```python
from build123d import *

# Parameters (mm, degrees)
BOSS_EXTRUDE1_DEPTH = 6.35
CUT_EXTRUDE1_REACH  = 8.35
SKETCH2_R           = 2.413
CUT_EXTRUDE3_REACH  = 8.35
SKETCH4_R           = 1.397
SKETCH4_R_2         = 4.7625
FILLET4_R           = 12.7
FILLET5_R           = 19.05


with BuildPart() as part:
    # Sketch1 → Boss-Extrude1 (new body)
    with BuildSketch(Plane.XY):
        Polygon((0, 0), (12.7, 0), (12.7, 50.8), (50.8, 50.8), (50.8, 0), (63.5, 0), (63.5, 69.85), (44.45, 101.6), (19.05, 101.6), (0, 82.55), align=None)
    extrude(amount=BOSS_EXTRUDE1_DEPTH)

    # Sketch2 → Cut-Extrude1 (cut, up to next)
    with BuildSketch(Plane.XY.offset(6.35), mode=Mode.PRIVATE) as cut_extrude1_sk1:
        with Locations((6.35, 12.7)):
            Circle(SKETCH2_R)
    cut_extrude1_tool1 = extrude(cut_extrude1_sk1.sketch, amount=-CUT_EXTRUDE1_REACH, mode=Mode.PRIVATE) & part.part
    add(cut_extrude1_tool1.solids().sort_by_distance((6.35, 12.7, 6.35))[0], mode=Mode.SUBTRACT)
    # Sketch2 → Cut-Extrude1 (cut, up to next)
    with BuildSketch(Plane.XY.offset(6.35), mode=Mode.PRIVATE) as cut_extrude1_sk2:
        with Locations((6.35, 31.75)):
            Circle(SKETCH2_R)
    cut_extrude1_tool2 = extrude(cut_extrude1_sk2.sketch, amount=-CUT_EXTRUDE1_REACH, mode=Mode.PRIVATE) & part.part
    add(cut_extrude1_tool2.solids().sort_by_distance((6.35, 31.75, 6.35))[0], mode=Mode.SUBTRACT)
    # Sketch2 → Cut-Extrude1 (cut, up to next)
    with BuildSketch(Plane.XY.offset(6.35), mode=Mode.PRIVATE) as cut_extrude1_sk3:
        with Locations((57.15, 12.7)):
            Circle(SKETCH2_R)
    cut_extrude1_tool3 = extrude(cut_extrude1_sk3.sketch, amount=-CUT_EXTRUDE1_REACH, mode=Mode.PRIVATE) & part.part
    add(cut_extrude1_tool3.solids().sort_by_distance((57.15, 12.7, 6.35))[0], mode=Mode.SUBTRACT)
    # Sketch2 → Cut-Extrude1 (cut, up to next)
    with BuildSketch(Plane.XY.offset(6.35), mode=Mode.PRIVATE) as cut_extrude1_sk4:
        with Locations((57.15, 31.75)):
            Circle(SKETCH2_R)
    cut_extrude1_tool4 = extrude(cut_extrude1_sk4.sketch, amount=-CUT_EXTRUDE1_REACH, mode=Mode.PRIVATE) & part.part
    add(cut_extrude1_tool4.solids().sort_by_distance((57.15, 31.75, 6.35))[0], mode=Mode.SUBTRACT)

    # Sketch4 → Cut-Extrude3 (cut, up to next)
    with BuildSketch(Plane.XY.offset(6.35), mode=Mode.PRIVATE) as cut_extrude3_sk1:
        with Locations((12.7, 52.3875)):
            Circle(SKETCH4_R)
    cut_extrude3_tool1 = extrude(cut_extrude3_sk1.sketch, amount=-CUT_EXTRUDE3_REACH, mode=Mode.PRIVATE) & part.part
    add(cut_extrude3_tool1.solids().sort_by_distance((12.7, 52.3875, 6.35))[0], mode=Mode.SUBTRACT)
    # Sketch4 → Cut-Extrude3 (cut, up to next)
    with BuildSketch(Plane.XY.offset(6.35), mode=Mode.PRIVATE) as cut_extrude3_sk2:
        with Locations((12.7, 87.3125)):
            Circle(SKETCH4_R)
    cut_extrude3_tool2 = extrude(cut_extrude3_sk2.sketch, amount=-CUT_EXTRUDE3_REACH, mode=Mode.PRIVATE) & part.part
    add(cut_extrude3_tool2.solids().sort_by_distance((12.7, 87.3125, 6.35))[0], mode=Mode.SUBTRACT)
    # Sketch4 → Cut-Extrude3 (cut, up to next)
    with BuildSketch(Plane.XY.offset(6.35), mode=Mode.PRIVATE) as cut_extrude3_sk3:
        with Locations((38.1, 69.85)):
            Circle(SKETCH4_R_2)
    cut_extrude3_tool3 = extrude(cut_extrude3_sk3.sketch, amount=-CUT_EXTRUDE3_REACH, mode=Mode.PRIVATE) & part.part
    add(cut_extrude3_tool3.solids().sort_by_distance((38.1, 69.85, 6.35))[0], mode=Mode.SUBTRACT)

    # Fillet4
    fillet4_edges = [part.edges().sort_by_distance(p)[0] for p in [
        (50.8, 50.8, 3.175),
        (12.7, 50.8, 3.175),
    ]]
    fillet(fillet4_edges, radius=FILLET4_R)

    # Fillet5
    fillet5_edges = [part.edges().sort_by_distance(p)[0] for p in [
        (0, 82.55, 3.175),
        (19.05, 101.6, 3.175),
        (44.45, 101.6, 3.175),
        (63.5, 69.85, 3.175),
    ]]
    fillet(fillet5_edges, radius=FILLET5_R)


solid = part.part
```
Check sheet for the modelled part. Datum: model origin and axes. Units: mm. A direction names the side the tool comes from. Coordinates: 2 decimals unless noted, no trailing zeros. Write each loop counter-clockwise with the first axis right and the second up, starting at its lowest first coordinate (ties: lowest second). Pieces come first, ordered by that corner, then holes. Notation, with made-up numbers: M 8.5,67.5 L 58.5,67.5 A27 cw 58.5,87.5 Z; hole C -15,-26 d6. An arc over 180 degrees is marked long. Write item = value, one per line. Start each with the question number.
1. Sectioned sample at C-C (y = 69.85). Record the cut outline in (x, z), then the cut area to 3 significant figures.
2. Sectioned sample at D-D (z = 2.75). State how many separate pieces and enclosed holes the cut face has, then the cut area to 3 significant figures.
3. Tool access check on faces 4 (the flat face through (50.8, 19, 3)), 5 (the flat face through (31, 52, 6.35)). Record the directions out of +Z, -Z, +X, -X, +Y, -Y that give a thin tool (end or side, any length) a straight path to the whole face; none if there is none.
4. Sectioned sample at B-B (x = 40.5). Record the cut outline in (y, z), then the cut area to 3 significant figures.
5. Sectioned sample at A-A (y = 12.7). Record the cut outline in (x, z), then the cut area to 4 significant figures.
6. Mould release check, pull along Y, two halves, no side actions. Record for faces 1 (the cylindrical face through (7.463, 10.559, 3.219)), 2 (the flat face through (0, 38, 3)), 3 (the cylindrical face through (19.55, 100.11, 3.22)): pulls with the +Y half, pulls with the -Y half, needs draft (parallel to the pull), parting line crosses it, or undercut.
7. Thickness scan on probe 1 along X at (y, z) = (32, 5.5); probe 2 along X at (y, z) = (44, 6); probe 3 along Y at (x, z) = (6, 2). Record the ranges inside material, lowest first.
8. Go/stop test with flat-tipped pins: pin 1 (2 mm diameter, centred on x = 12.7, y = 87.31, fed in from -Z); pin 2 (1.9 mm diameter, centred on x = 33.5, z = 3, fed in from -Y); pin 3 (2 mm diameter, centred on x = 6.5, z = 1.5, fed in from +Y). Record where each tip stops, or that it passes through.
The answers:
q1.outline = M 0,0 L 33.34,0 L 33.34,6.35 L 0,6.35 Z; M 42.86,0 L 62.75,0 L 62.75,6.35 L 42.86,6.35 Z
q1.area = 338 mm²
q2.separate_pieces = 1
q2.enclosed_holes = 7
q2.area = 3,910 mm²
q3.face_4 = +Z, -Z, -Y
q3.face_5 = +Z, +X, -X, +Y, -Y
q4.outline = M 50.57,0 L 65.74,0 L 65.74,6.35 L 50.57,6.35 Z; M 73.96,0 L 100.33,0 L 100.33,6.35 L 73.96,6.35 Z
q4.area = 264 mm²
q5.outline = M 0,0 L 3.94,0 L 3.94,6.35 L 0,6.35 Z; M 8.76,0 L 12.7,0 L 12.7,6.35 L 8.76,6.35 Z; M 50.8,0 L 54.74,0 L 54.74,6.35 L 50.8,6.35 Z; M 59.56,0 L 63.5,0 L 63.5,6.35 L 59.56,6.35 Z
q5.area = 100.0 mm²
q6.face_1 = undercut
q6.face_2 = needs draft
q6.face_3 = pulls with the +Y half
q7.probe_1 = 0 to 3.95, 8.75 to 12.7, 50.8 to 54.75, 59.55 to 63.5
q7.probe_2 = 0 to 14.15, 49.35 to 63.5
q7.probe_3 = 0 to 10.31, 15.09 to 29.36, 34.14 to 88.55
q8.pin_1 = through
q8.pin_2 = 50.8
q8.pin_3 = 90.05
